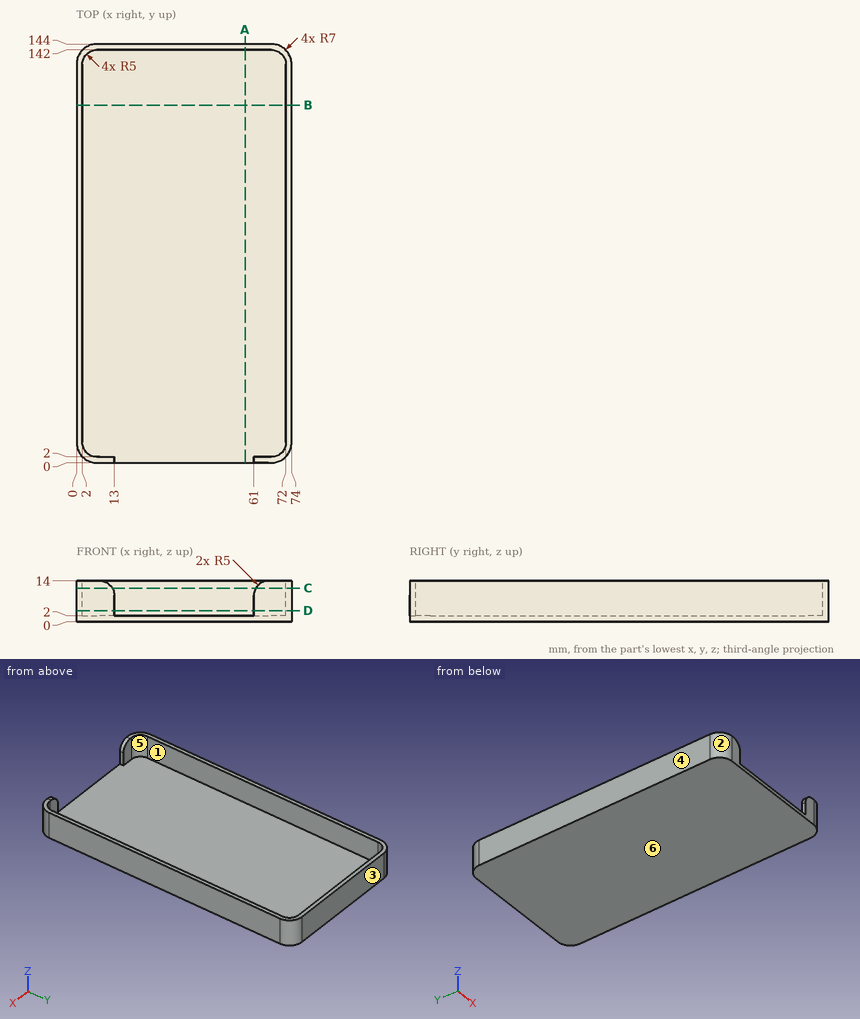
Input: dimensioned drawing with shaded views. Units: mm. Origin: part minimum x, y, z. A direction names the side the tool comes from. Coordinates: 2 decimals unless noted, no trailing zeros. Order: outer loops, then holes, each group sorted by start corner. A loop starts at its lowest first (then second) coordinate and runs counter-clockwise, first axis right, second up.
Item 1: Section query D-D (z = 3.75). Output: boundary loops of the cut face in (x, y), then the cut area to 3 significant figures.
Answer:
outline: (0, 7) arc R7 ccw to (7, 0) - (13, 0) - (13, 2) - (7, 2) arc R5 cw to (2, 7) - (2, 137) arc R5 cw to (7, 142) - (67, 142) arc R5 cw to (72, 137) - (72, 7) arc R5 cw to (67, 2) - (61, 2) - (61, 0) - (67, 0) arc R7 ccw to (74, 7) - (74, 137) arc R7 ccw to (67, 144) - (7, 144) arc R7 ccw to (0, 137) - close
area: 739 mm2
Item 2: Material intervals for line 1 along X through (y, z) = (30.5, 4); line 2 along Y through (x, z) = (65, 2.75); line 3 along Y through (x, z) = (20.5, 8.25), sorted ascending.
Answer:
line 1: x = 0 to 2, 72 to 74
line 2: y = 0 to 2, 142 to 144
line 3: y = 142 to 144
Item 3: Section query A-A (x = 58). Output: boundary loops of the cut face in (y, z).
Answer:
outline: (0, 0) - (144, 0) - (144, 14) - (142, 14) - (142, 2) - (0, 2) - close
Item 4: Draft query along Y for the marked faces 1, 2, 3 and 4. Return one class per face: released by +Y, released by -Y, zero draft, split by the parting line, or undercut.
Answer:
face 1: undercut
face 2: released by -Y
face 3: released by +Y
face 4: zero draft
Item 5: Section query B-B (y = 123). Output: boundary loops of the cut face in (x, z), then the cut area to 3 significant figures.
Answer:
outline: (0, 0) - (74, 0) - (74, 14) - (72, 14) - (72, 2) - (2, 2) - (2, 14) - (0, 14) - close
area: 196 mm2
Item 6: Access query for the marked faces 5 and 6. Directions: +Z, -Z, +X, -X, +Y, -Y. A direction counts if a zero-diameter tool reaches every point of the face in a straight line with its end or side. Return the directions, or none.
Answer:
face 5: +Z
face 6: -Z, +X, -X, +Y, -Y
Item 7: Section query C-C (z = 11.5). Output: boundary loops of the cut face in (x, y), then the cut area to 3 significant figures.
Answer:
outline: (0, 7) arc R7 ccw to (7, 0) - (12.33, 0) - (12.33, 2) - (7, 2) arc R5 cw to (2, 7) - (2, 137) arc R5 cw to (7, 142) - (67, 142) arc R5 cw to (72, 137) - (72, 7) arc R5 cw to (67, 2) - (61.67, 2) - (61.67, 0) - (67, 0) arc R7 ccw to (74, 7) - (74, 137) arc R7 ccw to (67, 144) - (7, 144) arc R7 ccw to (0, 137) - close
area: 737 mm2
Item 8: Contact query for flat-ended pins moving along their axis: P1, Ø2, axis at y = 1, z = 5.5, coming from the -X side; P2, Ø2, axis at y = 1, z = 7, coming from the +X side; P3, Ø10, axis at x = 46, y = 117.5, coming from the +Z side. Output: stop coordinate, or through.
Answer:
P1: stops at x = 2.1
P2: stops at x = 71.9
P3: stops at z = 2
